Autodesk Inventor part; units mm, degrees
ref_plane "YZ Plane" through (0, 0, 0) normal (1, 0, 0) x (0, 1, 0)
ref_plane "XZ Plane" through (0, 0, 0) normal (0, 1, 0) x (-1, 0, 0)
ref_plane "XY Plane" through (0, 0, 0) normal (0, 0, 1) x (1, 0, 0)
sketch "Sketch1" plane through (0, 0, 0) normal (0, 1, 0) x (-1, 0, 0)
  line L0 (5, 0) -> (165, 0)
  line L1 (170, -5) -> (170, -145)
  line L2 (165, -150) -> (5, -150)
  line L3 (0, -145) -> (0, -5)
  arc A0 (170, -5) -> (165, 0) centre (165, -5) ccw
  arc A1 (165, -150) -> (170, -145) centre (165, -145) ccw
  arc A2 (5, 0) -> (0, -5) centre (5, -5) ccw
  arc A3 (0, -145) -> (5, -150) centre (5, -145) ccw
  point P0 (0, 0)
  point P1 (170, -150)
  point P2 (170, 0)
  point P3 (0, -150)
  dimension "d0" = 170
  dimension "d1" = 150
  dimension "d2" = 5
extrude "Extrusion1" add sketch "Sketch1" along normal blind 12
sketch "Sketch2" plane through (0, 12, 0) normal (0, 1, 0) x (1, 0, 0)
  line L0 (0, 5) -> (0, 145)
  line L1 (-170, 145) -> (-170, 5)
  line L2 (-165, 0) -> (-5, 0)
  circle A0 centre (-85, 75) radius 20
  circle A1 centre (-85, 75) radius 30
  point P0 (0, 0)
  dimension "d5" = 40
  dimension "d6" = 60
extrude "Extrusion2" cut sketch "Sketch2" against normal blind 3
sketch "Sketch3" plane through (-85, 12, -75) normal (0, 1, 0) x (1, 0, 0)
  circle A0 centre (0, 0) radius 30
  circle A1 centre (0, 0) radius 20
  point P0 (85, -75)
extrude "Extrusion3" add sketch "Sketch3" along normal blind 3 contours A1
sketch "Sketch4" plane through (-85, 15, -75) normal (0, 1, 0) x (1, 0, 0)
  circle A0 centre (-12.5, 0) radius 1.75
  circle A1 centre (0, 12.5) radius 1.75
  circle A2 centre (0, -12.5) radius 1.75
  circle A3 centre (12.5, 0) radius 1.75
  point P0 (85, -75)
  dimension "d15" = 3.5
  dimension "d16" = 3.5
  dimension "d17" = 3.5
  dimension "d18" = 3.5
extrude "Extrusion4" cut sketch "Sketch4" against normal blind 20
sketch "Sketch5" plane through (0, 0, 0) normal (0, -1, 0) x (1, 0, 0)
  circle A0 centre (-85, -87.5) radius 1.75
  circle A1 centre (-85, -87.5) radius 3.5
  circle A2 centre (-72.5, -75) radius 1.75
  circle A3 centre (-72.5, -75) radius 3.5
  circle A4 centre (-85, -62.5) radius 1.75
  circle A5 centre (-85, -62.5) radius 3.5
  circle A6 centre (-97.5, -75) radius 1.75
  circle A7 centre (-97.5, -75) radius 3.5
  point P0 (0, 0)
  dimension "d21" = 7
  dimension "d22" = 7
  dimension "d23" = 7
  dimension "d24" = 7
extrude "Extrusion5" cut sketch "Sketch5" against normal blind 4
sketch "Sketch6" plane through (0, 0, 0) normal (0, -1, 0) x (1, 0, 0)
  line L0 (0, 0) -> (0, -20)
  line L1 (0, -5) -> (0, -145)
  line L2 (0, -20) -> (-15, -20)
  line L3 (0, -150) -> (0, -130)
  line L4 (0, -130) -> (-15, -130)
  line L5 (-170, 0) -> (-170, -20)
  line L6 (-170, -145) -> (-170, -5)
  line L7 (-170, -20) -> (-155, -20)
  line L8 (-170, -150) -> (-170, -130)
  line L9 (-170, -130) -> (-155, -130)
  circle A0 centre (-15, -20) radius 2.45
  circle A1 centre (-15, -130) radius 2.45
  circle A2 centre (-155, -20) radius 2.45
  circle A3 centre (-155, -130) radius 2.45
  dimension "d27" = 20
  dimension "d28" = 15
  dimension "d29" = 20
  dimension "d30" = 15
  dimension "d31" = 20
  dimension "d32" = 15
  dimension "d33" = 20
  dimension "d34" = 15
  dimension "d35" = 4.9
  dimension "d36" = 4.9
  dimension "d37" = 4.9
  dimension "d38" = 4.9
extrude "Extrusion6" cut sketch "Sketch6" against normal blind 15
properties part number "b_base_table"
The listing builds one solid part. Answer for the finished solid, in the listing's coordinates (mm). A direction names the side the tool comes from. Round coordinates to 2 decimals unless told otherwise and drop trailing zeros. Order: outer loops, then holes, each group sorted by start corner. A loop starts at its lowest first (then second) coordinate and runs counter-clockwise, first axis right, second up. Notation, with made-up numbers: (-14.75, -18.75) -> (-3.75, -18.75) arc R37 cw to (-3.75, 18.25) -> close; hole circle Ø2 at (43.25, -35). An arc over 180 degrees is marked (long way). Answer as CSV lines item,"result".
Q1. A cutting plane is placed at D-D on z = -108. Determine the outline of the cut face in (x, y), plus the area to 3 significant figures.
Computed values:
outline,"(-170, 0) -> (0, 0) -> (0, 12) -> (-170, 12) -> close"
area,"2,040 mm^2"
Q2. For a pull along Z with two mould halves and no side action, classify faces 3 (the cylindrical face through (-1, 6, -2)), 4 (the flat face through (-86, 6, -150)), 5 (the flat face through (-72, 4, -73)) as +Z half, -Z half, draft (parallel to the pull), parting line (faces both ways), or undercut.
Computed values:
face 3,"+Z half"
face 4,"-Z half"
face 5,"undercut"
Q3. Which of the six approach directions +Z, -Z, +X, -X, +Y, -Y give full straight-line access (tool end or side, diameter ignored) to faces 1 (the cylindrical face through (-81.767, 1.972, -88.841)), 2 (the flat face through (-84, 0, -74))?
Computed values:
face 1,"-Y"
face 2,"+Z, -Z, +X, -X, -Y"
Q4. Consider line 1 (X direction, y = 6.5, z = -130); line 2 (Z direction, x = -155, y = 4); line 3 (X direction, y = 12.75, z = -74). Determine where each line is inside the solid, lowest interval first. Write a range as from..to.
Computed values:
line 1,"x = -170..-157.45, -152.55..-17.45, -12.55..0"
line 2,"z = -150..-132.45, -127.55..-22.45, -17.55..0"
line 3,"x = -104.97..-98.94, -96.06..-73.94, -71.06..-65.03"
Q5. Given pin 1 (5.5 mm diameter, centred on x = -85, z = -63.5, fed in from -Y); pin 2 (4 mm diameter, centred on x = -72.5, z = -75, fed in from -Y); pin 3 (1.5 mm diameter, centred on x = -76, z = -100, fed in from +Y), each flat-ended and moving along its own axis, determine where each tip first touches the part or whether it passes through.
Computed values:
pin 1,"stops at y = 0"
pin 2,"stops at y = 4"
pin 3,"stops at y = 9"
Q6. A cutting plane is placed at C-C on x = -119.5. Determine the outline of the cut face in (y, z), plus the area to 3 significant figures.
Computed values:
outline,"(0, -150) -> (12, -150) -> (12, 0) -> (0, 0) -> close"
area,"1,800 mm^2"
Q7. A cutting plane is placed at B-B on x = -15. Determine the outline of the cut face in (y, z), plus the area to 3 significant figures.
Computed values:
outline,"(0, -150) -> (12, -150) -> (12, -132.45) -> (0, -132.45) -> close; (0, -127.55) -> (12, -127.55) -> (12, -22.45) -> (0, -22.45) -> close; (0, -17.55) -> (12, -17.55) -> (12, 0) -> (0, 0) -> close"
area,"1,680 mm^2"
Q8. A cutting plane is placed at A-A on z = -20. Determine the outline of the cut face in (x, y).
Computed values:
outline,"(-170, 0) -> (-157.45, 0) -> (-157.45, 12) -> (-170, 12) -> close; (-152.55, 0) -> (-17.45, 0) -> (-17.45, 12) -> (-152.55, 12) -> close; (-12.55, 0) -> (0, 0) -> (0, 12) -> (-12.55, 12) -> close"
